Can you work these out from the model? Positions are in its coordinate system, mm. A direction names the side the tool comes from. Give positions to 0.01 mm unless a question says otherwise; leave off trailing zeros. Order: outer loops, then holes, each group sorted by start corner. A loop starts at its lowest first (then second) coordinate and runs counter-clockwise, first axis right, second up. Notation, with made-up numbers: (86, -6) - (111, -6) arc R18 ccw to (111, 14) - close; hole circle Ø5 at (-35.75, 40). An arc over 180 degrees is marked (long way). One line per question, with ' | ' between items.
```python
from build123d import *

# Parameters (mm, degrees)
CROQUIS3_R            = 48.5
CORTAR_EXTRUIR1_DEPTH = 98.5
CROQUIS4_R            = 1.1
CORTAR_EXTRUIR2_DEPTH = 98.5
CROQUIS6_W            = 5.2
CROQUIS6_H            = 35.2
CORTAR_EXTRUIR3_DEPTH = 98.5
MATRIZC1_COUNT        = 12


with BuildPart() as part:
    # Croquis2 → Revolución2 (revolve)
    with BuildSketch(Plane.XY, mode=Mode.PRIVATE) as revoluci_n2_sk:
        Polygon((0, 0), (-10, 0), (-10, 5), (-50, 5), (-50, 105), (0, 105), align=None)
    revolve(revoluci_n2_sk.sketch.rotate(Axis((0, 0, 0), (0, 1, 0)), 270), axis=Axis((0, 0, 0), (0, 1, 0)))

    # Croquis3 → Cortar-Extruir1 (cut)
    with BuildSketch(Plane(origin=(0, 105, 0), x_dir=(1, 0, 0), z_dir=(0, 1, 0))):
        with Locations(Location((0, 0, 0), (0, 0, 270))):
            Circle(CROQUIS3_R)
    extrude(amount=-CORTAR_EXTRUIR1_DEPTH, mode=Mode.SUBTRACT)

    # Croquis4 → Cortar-Extruir2 (cut)
    with BuildSketch(Plane.XZ):
        with Locations(Location((0, 0, 0), (0, 0, 270))):
            Circle(CROQUIS4_R)
    extrude(amount=-CORTAR_EXTRUIR2_DEPTH, mode=Mode.SUBTRACT)

    # Croquis6 → Cortar-Extruir3 (cut)
    with BuildSketch(Plane.XY):
        with Locations((0, 67.4)):
            Rectangle(CROQUIS6_W, CROQUIS6_H)
    cortar_extruir3 = extrude(amount=-CORTAR_EXTRUIR3_DEPTH, mode=Mode.SUBTRACT)

    # MatrizC1: Cortar-Extruir3 ×12 about axis
    matrizc1_axis = Axis((0, 0, 0), (0, 1, 0))
    for i in range(1, MATRIZC1_COUNT):
        add(cortar_extruir3.rotate(matrizc1_axis, i * 360 / MATRIZC1_COUNT), mode=Mode.SUBTRACT)


solid = part.part
```
(1) Imagine slicing it at B-B (y = 41). List the corners of the cut face in (x, z) for me.
Answer below:
outline: circle Ø100 at (0, 0); hole circle Ø97 at (0, 0)
(2) Imagine slicing it at C-C (z = -18). List the corners of the cut face in (x, y) for me.
Answer below:
outline: (-46.65, 5) - (46.65, 5) - (46.65, 105) - (45.04, 105) - (45.04, 6.5) - (-45.04, 6.5) - (-45.04, 105) - (-46.65, 105) - close
(3) If we mould it in two halves opening along Z, with no side actions, what happens to faces 1 (the face through (-15.02, 55.7, -47.69)), 2 (the face through (-43, 49.8, 25)), 3 (the face through (0, 0, 2))? For each: released by +Z, released by -Z, zero draft, split by the parting line, or undercut.
Answer below:
face 1: split by the parting line | face 2: undercut | face 3: zero draft
(4) If I drill on line 1 (X direction, y = 3, z = 0); line 2 (Y direction, x = -38, z = -23.5); line 3 (Y direction, x = 2, z = -8.5), over which ranges is the centre line in solid material (lowest first)?
Answer below:
line 1: -10 to -1.1, 1.1 to 10 | line 2: 5 to 6.5 | line 3: 0 to 6.5
(5) Imagine slicing it at D-D (x = -38.5). List the corners of the cut face in (y, z) for me.
Answer below:
outline: (5, -31.9) - (105, -31.9) - (105, -29.5) - (6.5, -29.5) - (6.5, 29.5) - (105, 29.5) - (105, 31.9) - (5, 31.9) - close
(6) Imagine slicing it at A-A (x = -25). List the corners of the cut face in (y, z) for me.
Answer below:
outline: (5, -43.3) - (49.8, -43.3) - (49.8, -41.56) - (6.5, -41.56) - (6.5, 41.56) - (49.8, 41.56) - (49.8, 43.3) - (5, 43.3) - close; (85, -43.3) - (105, -43.3) - (105, -41.56) - (85, -41.56) - close; (85, 41.56) - (105, 41.56) - (105, 43.3) - (85, 43.3) - close
(7) Will these pins go through, and if not, where does the flat tip stop? pin 1 (12 mm diameter, centred on x = -10.5, y = 27.5, fed in from +Z); pin 2 (1 mm diameter, centred on x = 25.5, z = 17.5, fed in from -Y); pin 3 (1 mm diameter, centred on y = 90.5, z = 33.5, fed in from +X).
Answer below:
pin 1: z = 49.8 | pin 2: y = 5 | pin 3: x = 37.56
(8) On a 3-axis mill with a long thin cutter (end or side, diameter ignored), from which of +Z, -Z, +X, -X, +Y, -Y can I reach the whole of each face in a straight line? I mean faces 4 (the face through (-18.58, 56.44, 44.8)), 5 (the face through (9.76, 2.54, 2.17)), 6 (the face through (-41, 105, 26.2)). Say none if no direction works.
Answer below:
face 4: +Y | face 5: -Y | face 6: +Z, -Z, +X, -X, +Y
